Here's how the part is built. I have some questions about the finished solid (model axes, mm). A direction names the side the tool comes from. Coordinates: 2 decimals unless noted, no trailing zeros. Order: outer loops, then holes, each group sorted by start corner. A loop starts at its lowest first (then second) coordinate and runs counter-clockwise, first axis right, second up. Notation, with made-up numbers: M 75,47 L 102,47 A5 ccw 102,56 Z; hole C -15,-9 d11. An arc over 180 degrees is marked long. Answer as CSV lines item,"result". Start each with the question number.
```python
from build123d import *

# Parameters (mm, degrees)
BASEFLANGE_W                   = 920
BASEFLANGE_H                   = 50
BASE_FLANGE1_DEPTH             = 2
EDGE_FLANGE1_STRIP_W           = 10
EDGE_FLANGE1_STRIP_H           = 2
EDGE_FLANGE1_STRIP_CUT_DEPTH   = 920
EDGE_FLANGE1_DEPTH             = 920
EDGE_FLANGE2_STRIP_W           = 10
EDGE_FLANGE2_STRIP_H           = 2
EDGE_FLANGE2_STRIP_CUT_DEPTH   = 47
EDGE_FLANGE2_STRIP_2_W         = 10
EDGE_FLANGE2_STRIP_2_H         = 2
EDGE_FLANGE2_STRIP_CUT_2_DEPTH = 47
EDGE_FLANGE2_DEPTH             = 47
EDGE_FLANGE2_BEND_DEPTH        = 47


# Sheet-metal steps are written as plain solids
with BuildPart() as part:
    # BaseFlange → Base-Flange1 (new body)
    with BuildSketch(Plane.XY):
        with Locations((0, -25)):
            Rectangle(BASEFLANGE_W, BASEFLANGE_H)
    extrude(amount=BASE_FLANGE1_DEPTH)

    # Edge-Flange1 strip (across the edge) → Edge-Flange1 strip cut (cut)
    with BuildSketch(Plane(origin=(460, 0, 2), x_dir=(0, -1, 0), z_dir=(-1, 0, 0))):
        with Locations((-2, -1)):
            Rectangle(EDGE_FLANGE1_STRIP_W, EDGE_FLANGE1_STRIP_H)
    extrude(amount=EDGE_FLANGE1_STRIP_CUT_DEPTH, mode=Mode.SUBTRACT)

    # Edge-Flange1 section (across the edge) → Edge-Flange1 (add)
    with BuildSketch(Plane(origin=(460, 0, 2), x_dir=(0, -1, 0), z_dir=(-1, 0, 0))):
        with BuildLine():
            Line((0, 1), (0, 48))
            Line((0, 48), (2, 48))
            Line((2, 48), (2, 1))
            ThreePointArc((2, 1), (2.292893219, 0.292893219), (3, 0))
            Line((3, 0), (3, -2))
            ThreePointArc((3, -2), (0.878679656, -1.121320344), (0, 1))
        make_face()
    extrude(amount=EDGE_FLANGE1_DEPTH)

    # Edge-Flange2 strip (across the edge) → Edge-Flange2 strip cut (cut)
    with BuildSketch(Plane(origin=(460, -50, 2), x_dir=(-1, 0, 0), z_dir=(0, 1, 0))):
        with Locations((-2, -1)):
            Rectangle(EDGE_FLANGE2_STRIP_W, EDGE_FLANGE2_STRIP_H)
    extrude(amount=EDGE_FLANGE2_STRIP_CUT_DEPTH, mode=Mode.SUBTRACT)

    # Edge-Flange2 strip 2 (across the edge) → Edge-Flange2 strip cut 2 (cut)
    with BuildSketch(Plane(origin=(-460, -3, 2), x_dir=(1, 0, 0), z_dir=(0, -1, 0))):
        with Locations((-2, -1)):
            Rectangle(EDGE_FLANGE2_STRIP_2_W, EDGE_FLANGE2_STRIP_2_H)
    extrude(amount=EDGE_FLANGE2_STRIP_CUT_2_DEPTH, mode=Mode.SUBTRACT)

    # Edge-Flange2 section (across the edge) → Edge-Flange2 (add)
    with BuildSketch(Plane(origin=(460, -50, 2), x_dir=(-1, 0, 0), z_dir=(0, 1, 0))):
        with BuildLine():
            Line((0, 1), (0, 13))
            Line((0, 13), (2, 13))
            Line((2, 13), (2, 1))
            ThreePointArc((2, 1), (2.292893219, 0.292893219), (3, 0))
            Line((3, 0), (3, -2))
            ThreePointArc((3, -2), (0.878679656, -1.121320344), (0, 1))
        make_face()
    extrude(amount=EDGE_FLANGE2_DEPTH)

    # Edge-Flange2 section 2 (across the edge) → Edge-Flange2 bend (add)
    with BuildSketch(Plane(origin=(-460, -3, 2), x_dir=(1, 0, 0), z_dir=(0, -1, 0))):
        with BuildLine():
            Line((0, 1), (0, 13))
            Line((0, 13), (2, 13))
            Line((2, 13), (2, 1))
            ThreePointArc((2, 1), (2.292893219, 0.292893219), (3, 0))
            Line((3, 0), (3, -2))
            ThreePointArc((3, -2), (0.878679656, -1.121320344), (0, 1))
        make_face()
    extrude(amount=EDGE_FLANGE2_BEND_DEPTH)


solid = part.part
```
1) Which directions (+Z, -Z, +X, -X, +Y, -Y) give clear straight access to the entire face, cutting with the end or side of a thin tool? Please do faces 1 (the face through (2, -50, 1)), 2 (the face through (-6, -26, 2)).
2) Will these pins go through, and if not, where does the flat tip stop? pin 1 Ø14 at (x, z) = (115.5, 29) entering from -Y; pin 2 Ø14 at (x, y) = (194.5, -22) entering from +Z; pin 3 Ø1 at (x, y) = (-459, -26) entering from +Z; pin 4 Ø8 at (x, y) = (49, -37) entering from -Z.
3) I need wall thicknesses on line 1 (X direction, y = -46, z = 14); line 2 (Z direction, x = 417, y = -19); line 3 (Y direction, x = 252.5, z = 10). Which ranges of each line are inside material? Lowest first, please. Write a range as [from, to].
4) Suppose I cut it at A-A on y = -27. Please give me the cut outline in (x, z).
5) Suppose I cut it at C-C on z = 28. Please give me the cut outline in (x, y), plus the area to 3 significant figures.
6) Suppose I cut it at B-B on x = -396. Please give me the cut outline in (y, z), plus the area to 3 significant figures.
Output:
1,face 1,"+Z, -Z, +X, -X, -Y"
1,face 2,"+Z, -Y"
2,pin 1,"y = -2"
2,pin 2,"z = 2"
2,pin 3,"z = 15"
2,pin 4,"z = 0"
3,line 1,"[-460, -458], [458, 460]"
3,line 2,"[0, 2]"
3,line 3,"[-2, 0]"
4,outline,"M -460,3 A3 ccw -457,0 L 457,0 A3 ccw 460,3 L 460,15 L 458,15 L 458,3 A1 cw 457,2 L -457,2 A1 cw -458,3 L -458,15 L -460,15 Z"
5,outline,"M -460,-2 L 460,-2 L 460,0 L -460,0 Z"
5,area,"1,840 mm²"
6,outline,"M -50,0 L -3,0 A3 ccw 0,3 L 0,50 L -2,50 L -2,3 A1 cw -3,2 L -50,2 Z"
6,area,"194 mm²"
